Can you work these out from the model? Positions are in its coordinate system, mm. Face numbers are marked on the shaded views. A direction names the side the tool comes from. Coordinates: 2 decimals unless noted, no trailing zeros. Order: outer loops, then holes, each group sorted by start corner. A loop starts at its lowest first (then second) coordinate and runs counter-clockwise, first axis right, second up. Notation, with made-up numbers: (20.25, 38.25) -> (44.25, 38.25) arc R22 cw to (44.25, 76.25) -> close; hole circle Ø9 at (-34, 14.25). An arc over 180 degrees is marked (long way). Use a Markdown table: item, result. Add a question column.
1. For the marked faces 1, 2, 3 and 4, which set-ups out of +Z, -Z, +X, -X, +Y, -Y let a thin tool reach every point of the face, with its end or its side?
2. If I drill on line 1 along Y through (x, z) = (-43, 2.7); line 2 along Y through (x, z) = (-37.5, 2); line 3 along Y through (x, z) = (-48.25, -2), over which ranges is the centre line in solid material (lowest first)? Write a range as from..to.
3. For pin 1 Ø3.5 at (x, y) = (-34, 0) entering from -Z; pin 2 Ø6 at (x, y) = (-43.5, -21.5) entering from -Z, each with a flat end and sliding along its axis, tell me the tip position at first contact or that it passes through.
4. We'd pull the mould along X, two halves only. Please class the marked faces 5 and 6: pulls with the +X half, pulls with the -X half, needs draft (parallel to the pull), parting line crosses it, or undercut.
5. Suppose I cut it at B-B, the plane z = -9. List the corners of the cut face in (x, y) for me.
6. Suppose I cut it at A-A, the plane y = -5.5. List the corners of the cut face in (x, z) for me.
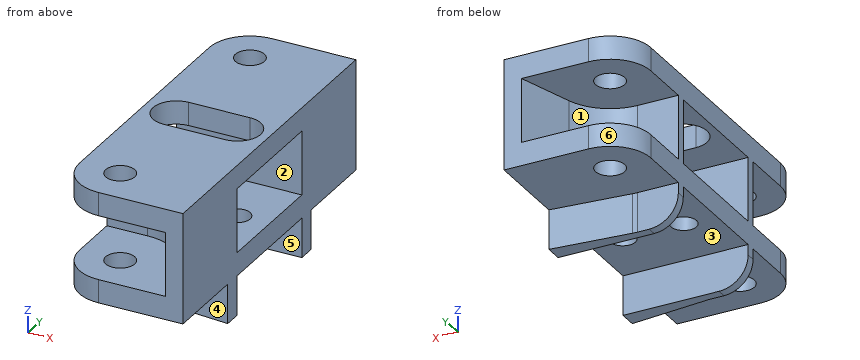
```python
from build123d import *

# Parameters (mm, degrees)
SKETCH_1_R      = 2.5
EXTRUDE_1_DEPTH = 4
EXTRUDE_2_DEPTH = 11
EXTRUDE_START   = -15
SKETCH_1_6_R    = 2.5
SKETCH_1_6_R_2  = 2.2
EXTRUDE_3_DEPTH = 4
EXTRUDE_4_DEPTH = 6.8
FILLET_1_R      = 5


with BuildPart() as part:
    # 草图1 → 凸台-拉伸1 (new body)
    with BuildSketch(Plane.XY):
        with BuildLine():
            ThreePointArc((-43, 28), (-47.949747468, 25.949747468), (-50, 21))
            Line((-50, 21), (-50, -21))
            ThreePointArc((-50, -21), (-47.949747468, -25.949747468), (-43, -28))
            Line((-43, -28), (-28.5, -28))
            Line((-28.5, -28), (-28.5, 28))
            Line((-28.5, 28), (-43, 28))
        make_face()
        with Locations((-43, 21)):
            Circle(SKETCH_1_R, mode=Mode.SUBTRACT)
        with BuildLine():
            Line((-44.5, 4), (-34, 4))
            ThreePointArc((-34, 4), (-30, 0), (-34, -4))
            Line((-34, -4), (-44.5, -4))
            ThreePointArc((-44.5, -4), (-48.5, 0), (-44.5, 4))
        make_face(mode=Mode.SUBTRACT)
        with Locations((-43, -21)):
            Circle(SKETCH_1_R, mode=Mode.SUBTRACT)
    extrude(amount=EXTRUDE_1_DEPTH)

    # 草图1<5> → 凸台-拉伸2 (add)
    with BuildSketch(Plane.XY):
        with BuildLine():
            Line((-43, 12.1), (-50, 12.1))
            Line((-50, 12.1), (-50, 10.5))
            Line((-50, 10.5), (-28.5, 10.5))
            Line((-28.5, 10.5), (-28.5, 28))
            Line((-28.5, 28), (-31.5, 28))
            Line((-31.5, 28), (-34.502137832, 18.354940724))
            ThreePointArc((-34.502137832, 18.354940724), (-37.724160141, 13.832328567), (-43, 12.1))
        make_face()
        with BuildLine():
            Line((-28.5, -10.5), (-50, -10.5))
            Line((-50, -10.5), (-50, -12.1))
            Line((-50, -12.1), (-43, -12.1))
            ThreePointArc((-43, -12.1), (-37.724160141, -13.832328567), (-34.502137832, -18.354940724))
            Line((-34.502137832, -18.354940724), (-31.5, -28))
            Line((-31.5, -28), (-28.5, -28))
            Line((-28.5, -28), (-28.5, -10.5))
        make_face()
    extrude(amount=-EXTRUDE_2_DEPTH)

    # 草图1<6> → 凸台-拉伸3 (add)
    with BuildSketch(Plane.XY.offset(EXTRUDE_START)):
        with BuildLine():
            ThreePointArc((-43, 28), (-47.949747468, 25.949747468), (-50, 21))
            Line((-50, 21), (-50, -21))
            ThreePointArc((-50, -21), (-47.949747468, -25.949747468), (-43, -28))
            Line((-43, -28), (-28.5, -28))
            Line((-28.5, -28), (-28.5, 28))
            Line((-28.5, 28), (-43, 28))
        make_face()
        with Locations((-43, 21)):
            Circle(SKETCH_1_6_R, mode=Mode.SUBTRACT)
        with Locations((-43, -21)):
            Circle(SKETCH_1_6_R, mode=Mode.SUBTRACT)
        with Locations((-34, 0)):
            Circle(SKETCH_1_6_R_2, mode=Mode.SUBTRACT)
        with Locations((-44.5, 0)):
            Circle(SKETCH_1_6_R_2, mode=Mode.SUBTRACT)
    extrude(amount=EXTRUDE_3_DEPTH)

    # 草图1<7> → 凸台-拉伸4 (add)
    with BuildSketch(Plane.XY.offset(EXTRUDE_START)):
        with BuildLine():
            Line((-43, 12.1), (-50, 12.1))
            Line((-50, 12.1), (-50, 10.5))
            Line((-50, 10.5), (-28.5, 10.5))
            Line((-28.5, 10.5), (-28.5, 13.5))
            Line((-28.5, 13.5), (-42.118030123, 12.143808429))
            ThreePointArc((-42.118030123, 12.143808429), (-42.558471393, 12.110958854), (-43, 12.1))
        make_face()
        with BuildLine():
            Line((-28.5, -10.5), (-50, -10.5))
            Line((-50, -10.5), (-50, -12.1))
            Line((-50, -12.1), (-43, -12.1))
            ThreePointArc((-43, -12.1), (-42.558471393, -12.110958854), (-42.118030123, -12.143808429))
            Line((-42.118030123, -12.143808429), (-28.5, -13.5))
            Line((-28.5, -13.5), (-28.5, -10.5))
        make_face()
    extrude(amount=-EXTRUDE_4_DEPTH)

    # 圆角1
    fillet_1_edges = [part.edges().sort_by_distance(p)[0] for p in [
        (-50, 11.3, -21.8),
        (-50, -11.3, -21.8),
    ]]
    fillet(fillet_1_edges, radius=FILLET_1_R)


solid = part.part
```
Worked out:
| question | item | result |
|---|---|---|
| 1 | face 1 | -X, +Y |
| 1 | face 2 | +X, -X |
| 1 | face 3 | -Z, +X, -X |
| 1 | face 4 | -Z, -X, -Y |
| 2 | line 1 | y = -28..-23.5, -18.5..-4, 4..18.5, 23.5..28 |
| 2 | line 2 | y = -28..-4, 4..28 |
| 2 | line 3 | y = -12.1..-10.5, 10.5..12.1 |
| 3 | pin 1 | passes through |
| 3 | pin 2 | stops at z = -15 |
| 4 | face 5 | needs draft |
| 4 | face 6 | pulls with the -X half |
| 5 | outline | (-50, -12.1) -> (-43, -12.1) arc R8.9 cw to (-34.5, -18.35) -> (-31.5, -28) -> (-28.5, -28) -> (-28.5, -10.5) -> (-50, -10.5) -> close; (-50, 10.5) -> (-28.5, 10.5) -> (-28.5, 28) -> (-31.5, 28) -> (-34.5, 18.35) arc R8.9 cw to (-43, 12.1) -> (-50, 12.1) -> close |
| 6 | outline | (-50, -15) -> (-28.5, -15) -> (-28.5, -11) -> (-50, -11) -> close; (-50, 0) -> (-28.5, 0) -> (-28.5, 4) -> (-50, 4) -> close |
